from build123d import *

# Parameters (mm, degrees)
SKETCH1_R           = 8.4
SKETCH1_R_2         = 3.4
BOSS_EXTRUDE1_DEPTH = 20
SKETCH2_R           = 8.4
SKETCH2_R_2         = 2.4
BOSS_EXTRUDE2_DEPTH = 1.5
SKETCH3_R           = 15
SKETCH3_R_2         = 10
BOSS_EXTRUDE3_DEPTH = 5
SKETCH5_R           = 28
SKETCH5_R_2         = 10
BOSS_EXTRUDE4_DEPTH = 5
CUT_EXTRUDE1_DEPTH  = 5


with BuildPart() as part:
    # Sketch1 → Boss-Extrude1 (new body)
    with BuildSketch(Plane.XY):
        Circle(SKETCH1_R)
        Circle(SKETCH1_R_2, mode=Mode.SUBTRACT)
    extrude(amount=BOSS_EXTRUDE1_DEPTH)

    # Sketch2 → Boss-Extrude2 (add)
    with BuildSketch(Plane.XY.offset(20)):
        Circle(SKETCH2_R)
        Circle(SKETCH2_R_2, mode=Mode.SUBTRACT)
    extrude(amount=-BOSS_EXTRUDE2_DEPTH)



with BuildPart() as body_2:
    # Sketch3 → Boss-Extrude3 (new body)
    with BuildSketch(Plane.XY.offset(35)):
        Circle(SKETCH3_R)
        Circle(SKETCH3_R_2, mode=Mode.SUBTRACT)
    extrude(amount=BOSS_EXTRUDE3_DEPTH)


with BuildPart() as part_1:
    add(part.part)

    add(body_2.part)  # Revolve1 merges body 2
    # Sketch4 → Revolve1 (revolve)
    with BuildSketch(Plane(origin=(0, 0, 0), x_dir=(1, 0, 0), z_dir=(0, 1, 0))):
        Polygon((-8.4, -20), (-15, -35), (-10, -35), (-2.4, -20), align=None)
    revolve(axis=Axis((0, 0, 20), (0, 0, 1)))

    # Sketch5 → Boss-Extrude4 (add)
    with BuildSketch(Plane.XY.offset(40)):
        Circle(SKETCH5_R)
        Circle(SKETCH5_R_2, mode=Mode.SUBTRACT)
    extrude(amount=-BOSS_EXTRUDE4_DEPTH)

    # Sketch6 → Cut-Extrude1 (cut)
    with BuildSketch(Plane(origin=(0, 0, 35), x_dir=(-1, 0, 0), z_dir=(0, 0, -1))):
        with BuildLine():
            Line((-1.55, 24), (-1.55, 29))
            Line((-1.55, 29), (1.55, 29))
            Line((1.55, 29), (1.55, 24))
            ThreePointArc((1.55, 24), (0, 22.45), (-1.55, 24))
        make_face()
        with BuildLine():
            Line((21.602112165, 19.410081144), (18.066578259, 15.874547238))
            ThreePointArc((18.066578259, 15.874547238), (15.874547238, 15.874547238), (15.874547238, 18.066578259))
            Line((15.874547238, 18.066578259), (19.410081144, 21.602112165))
            Line((19.410081144, 21.602112165), (21.602112165, 19.410081144))
        make_face()
        with BuildLine():
            Line((29, -1.55), (24, -1.55))
            ThreePointArc((24, -1.55), (22.45, 0), (24, 1.55))
            Line((24, 1.55), (29, 1.55))
            Line((29, 1.55), (29, -1.55))
        make_face()
        with BuildLine():
            Line((19.410081144, -21.602112165), (15.874547238, -18.066578259))
            ThreePointArc((15.874547238, -18.066578259), (15.874547238, -15.874547238), (18.066578259, -15.874547238))
            Line((18.066578259, -15.874547238), (21.602112165, -19.410081144))
            Line((21.602112165, -19.410081144), (19.410081144, -21.602112165))
        make_face()
        with BuildLine():
            Line((-1.55, -29), (-1.55, -24))
            ThreePointArc((-1.55, -24), (0, -22.45), (1.55, -24))
            Line((1.55, -24), (1.55, -29))
            Line((1.55, -29), (-1.55, -29))
        make_face()
        with BuildLine():
            Line((-21.602112165, -19.410081144), (-18.066578259, -15.874547238))
            ThreePointArc((-18.066578259, -15.874547238), (-15.874547238, -15.874547238), (-15.874547238, -18.066578259))
            Line((-15.874547238, -18.066578259), (-19.410081144, -21.602112165))
            Line((-19.410081144, -21.602112165), (-21.602112165, -19.410081144))
        make_face()
        with BuildLine():
            Line((-29, 1.55), (-24, 1.55))
            ThreePointArc((-24, 1.55), (-22.45, 0), (-24, -1.55))
            Line((-24, -1.55), (-29, -1.55))
            Line((-29, -1.55), (-29, 1.55))
        make_face()
        with BuildLine():
            Line((-19.410081144, 21.602112165), (-15.874547238, 18.066578259))
            ThreePointArc((-15.874547238, 18.066578259), (-15.874547238, 15.874547238), (-18.066578259, 15.874547238))
            Line((-18.066578259, 15.874547238), (-21.602112165, 19.410081144))
            Line((-21.602112165, 19.410081144), (-19.410081144, 21.602112165))
        make_face()
    extrude(amount=-CUT_EXTRUDE1_DEPTH, mode=Mode.SUBTRACT)


solid = part_1.part
Can you work these out from the model? Positions are in its coordinate system, mm. A direction names the side the tool comes from. Give positions to 0.01 mm unless a question says otherwise; leave off trailing zeros. Write each loop counter-clockwise with the first axis right and the second up, starting at its lowest first coordinate (ties: lowest second). Pieces come first, ordered by that corner, then holes. Notation, with made-up numbers: (79, 87.25) -> (130, 87.25) arc R33 cw to (130, 118.25) -> close; hole circle Ø9 at (41.5, 68). An arc over 180 degrees is marked (long way). Answer as a JSON object with one key per item and string values. Group by question number.
Item 1: We'd pull the mould along X, two halves only. Please class faces 1 (the face through (15.9, -15.85, 37.47)), 2 (the face through (8.012, 2.523, 9.86)), 3 (the face through (-26, -1.55, 37)): +X half, -X half, draft (parallel to the pull), parting line (faces both ways), or undercut.
Item 2: I'm going to push flat-ended pins straight in: P1, Ø3, axis at y = -9, z = 6, coming from the -X side; P2, Ø4, axis at y = -7, z = 7.5, coming from the +X side; P3, Ø4, axis at x = -10, y = -7, coming from the -Z side. Where does each tip first touch, or does it pass through?
Item 3: Suppose I cut it at D-D (z = 25). Please give me the cut outline in (x, y).
Item 4: Suppose I cut it at C-C (z = 10.5). Please give me the cut outline in (x, y), plus the area to 3 significant figures.
Item 5: For faces 4 (the face through (-19.485, 17.293, 37.465)), 5 (the face through (-2.17, -9.76, 37.47)), 6 (the face through (1.55, -26, 37)), which set-ups out of +Z, -Z, +X, -X, +Y, -Y let a thin tool reach every point of the face, with its end or its side?
Item 6: Please list where these lines run through material, in increasing order: line 1 (Y direction, x = 0, z = 9.75); line 2 (Y direction, x = 0, z = 19). Write a range as [from, to].
Item 7: Suppose I cut it at A-A (x = 0). Please give me the cut outline in (y, z).
Findings:
{
 "1": {"face 1": "undercut", "face 2": "parting line", "face 3": "draft"},
 "2": {"P1": "stops at x = -3.78", "P2": "stops at x = 6.75", "P3": "stops at z = 24.11"},
 "3": {"outline": "circle Ø21.2 at (0, 0); hole circle Ø9.87 at (0, 0)"},
 "4": {"outline": "circle Ø16.8 at (0, 0); hole circle Ø6.8 at (0, 0)", "area": "185 mm²"},
 "5": {"face 4": "+Z, -Z", "face 5": "+Z", "face 6": "+Z, -Z, -Y"},
 "6": {"line 1": "y = [-8.4, -3.4], [3.4, 8.4]", "line 2": "y = [-8.4, -2.4], [2.4, 8.4]"},
 "7": {"outline": "(-22.45, 35) -> (-15, 35) -> (-8.4, 20) -> (-8.4, 0) -> (-3.4, 0) -> (-3.4, 18.5) -> (-2.4, 18.5) -> (-2.4, 20) -> (-10, 35) -> (-10, 40) -> (-22.45, 40) -> close; (2.4, 18.5) -> (3.4, 18.5) -> (3.4, 0) -> (8.4, 0) -> (8.4, 20) -> (15, 35) -> (22.45, 35) -> (22.45, 40) -> (10, 40) -> (10, 35) -> (2.4, 20) -> close"}
}
